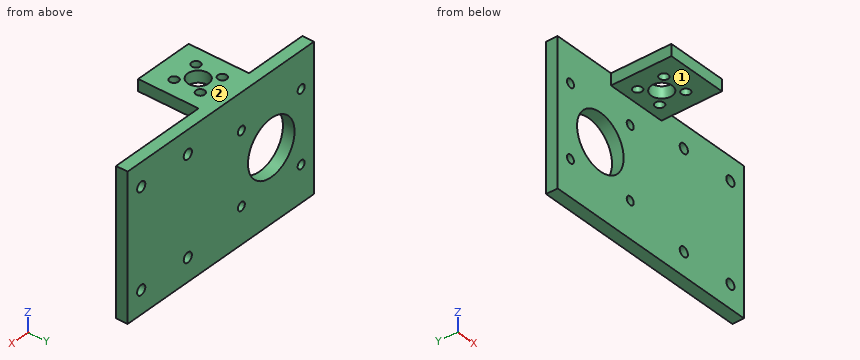
```python
from build123d import *

# Parameters (mm, degrees)
F0_W     = 96
F0_H     = 62
F0_R     = 1.8
F0_R_2   = 2.1
F0_R_3   = 12
F1_DEPTH = 5
F2_W     = 26
F2_H     = 5
F3_DEPTH = 26
F4_R     = 4.5
F4_R_2   = 1.8935291465
F5_DEPTH = 25


# Not quite as in the source:
# - a feature names something its author has since deleted; it is built from what else it names


with BuildPart() as f1:
    # F0 (on Front) → F1 (new body)
    with BuildSketch(Plane.XZ):
        with Locations((0, 31)):
            Rectangle(F0_W, F0_H)
        with Locations((-41.4, 15.6001571745)):
            Circle(F0_R, mode=Mode.SUBTRACT)
        with Locations((-10.6, 15.6001571745)):
            Circle(F0_R, mode=Mode.SUBTRACT)
        with Locations((17, 10)):
            Circle(F0_R_2, mode=Mode.SUBTRACT)
        with Locations((41, 10)):
            Circle(F0_R_2, mode=Mode.SUBTRACT)
        with Locations((-26, 31)):
            Circle(F0_R_3, mode=Mode.SUBTRACT)
        with Locations((-41.4, 46.4001571745)):
            Circle(F0_R, mode=Mode.SUBTRACT)
        with Locations((-10.6, 46.4001571745)):
            Circle(F0_R, mode=Mode.SUBTRACT)
        with Locations((17, 52)):
            Circle(F0_R_2, mode=Mode.SUBTRACT)
        with Locations((41, 52)):
            Circle(F0_R_2, mode=Mode.SUBTRACT)
    extrude(amount=F1_DEPTH)

    # F2 (on face) → F3 (join)
    with BuildSketch(Plane.XZ.offset(5)):
        with Locations((-7.5, 59.5)):
            Rectangle(F2_W, F2_H)
    extrude(amount=F3_DEPTH)

    # F4 (on face) → F5 (cut)
    with BuildSketch(Plane.XY.offset(62)):
        with Locations((-7.5, -16)):
            Circle(F4_R)
        with Locations((-13.1568542495, -10.3431457505)):
            Circle(F4_R_2)
        with Locations((-1.8431457505, -10.3431457505)):
            Circle(F4_R_2)
        with Locations((-1.8431457505, -21.6568542495)):
            Circle(F4_R_2)
        with Locations((-13.1568542495, -21.6568542495)):
            Circle(F4_R_2)
    extrude(amount=-F5_DEPTH, mode=Mode.SUBTRACT)


solid = f1.part
```
Design review of the part built by this model. Coordinates are the model's own, in mm. Face numbers are marked on the shaded views. A direction names the side the tool comes from. Round coordinates to 2 decimals unless told otherwise and drop trailing zeros. Order: outer loops, then holes, each group sorted by start corner. A loop starts at its lowest first (then second) coordinate and runs counter-clockwise, first axis right, second up. Notation, with made-up numbers: (-19, -20) - (-2, -20) arc R21 cw to (-2, 19) - close; hole circle Ø2 at (16.5, 6). An arc over 180 degrees is marked (long way). Return JSON: item names as keys, results as strings.
Q1. Machinability: for the marked faces 1 and 2, which of the approach directions +Z, -Z, +X, -X, +Y, -Y give a long, thin tool a straight path to every point of the face, cutting with its end or side? Answer none if there is none.
Computed values:
{"face 1": "-Z, +X, -X, -Y", "face 2": "+Z, +X, -X, +Y, -Y"}
Q2. Consider section B-B on x = 41. Write out the cut boundary in (y, z), plus the area to 3 significant figures.
Computed values:
{"outline": "(-5, 0) - (0, 0) - (0, 7.9) - (-5, 7.9) - close; (-5, 12.1) - (0, 12.1) - (0, 49.9) - (-5, 49.9) - close; (-5, 54.1) - (0, 54.1) - (0, 62) - (-5, 62) - close", "area": "268 mm2"}
Q3. Wall thickness on L1, parallel to Z at x = -41.4, y = -3.3; L2, parallel to Z at x = 41, y = -2.1; L3, parallel to Y at x = -42.5, z = 38: over which ranges is each line inside the solid? List them lowest first. Write a range as [from, to].
Computed values:
{"L1": "z = [0, 13.8], [17.4, 44.6], [48.2, 62]", "L2": "z = [0, 7.9], [12.1, 49.9], [54.1, 62]", "L3": "y = [-5, 0]"}
Q4. Consider section D-D on x = -7.5. Write out the cut boundary in (y, z).
Computed values:
{"outline": "(-31, 57) - (-20.5, 57) - (-20.5, 62) - (-31, 62) - close; (-11.5, 57) - (-5, 57) - (-5, 0) - (0, 0) - (0, 62) - (-11.5, 62) - close"}
Q5. For pin 1 Ø4 at (x, z) = (-41.4, 15.6) entering from -Y; pin 2 Ø4.5 at (x, y) = (-1.84, -10.34) entering from -Z; pin 3 Ø5.5 at (y, z) = (-18, 60.5) entering from -X, all flat-tipped, find the tip position at first contact; note any pin that passes through.
Computed values:
{"pin 1": "stops at y = -5", "pin 2": "stops at z = 57", "pin 3": "stops at x = -20.5"}
Q6. Consider section C-C on z = 36. Write out the cut boundary in (x, y), plus the area to 3 significant figures.
Computed values:
{"outline": "(-48, -5) - (-36.91, -5) - (-36.91, 0) - (-48, 0) - close; (-15.09, -5) - (48, -5) - (48, 0) - (-15.09, 0) - close", "area": "371 mm2"}
Q7. Consider section A-A on y = -16. Write out the cut boundary in (x, z), plus the area to 3 significant figures.
Computed values:
{"outline": "(-20.5, 57) - (-12, 57) - (-12, 62) - (-20.5, 62) - close; (-3, 57) - (5.5, 57) - (5.5, 62) - (-3, 62) - close", "area": "85.0 mm2"}
